Autodesk Inventor part; units mm, degrees
ref_plane "Work Plane1" through (0, 4.7752, 0) normal (0, -1, 0) x (1, 0, 0)
ref_plane "YZ Plane" through (0, 0, 0) normal (1, 0, 0) x (0, 1, 0)
ref_plane "XZ Plane" through (0, 0, 0) normal (0, 1, 0) x (-1, 0, 0)
sketch "Sketch2" plane through (0, 0, 0) normal (0, 1, 0) x (-1, 0, 0)
  line L0 (23, 23) -> (-23, 23)
  line L1 (-23, 23) -> (-23, -23)
  line L2 (-23, -23) -> (23, -23)
  line L3 (23, -23) -> (23, 23)
  line L4 (23, 23) -> (-23, -23) construction
  line L5 (-23, 23) -> (23, -23) construction
  circle A0 centre (19.05, -19.05) radius 1.8669
  line L6 (0, -32.2) -> (0, 32.2) construction
  line L7 (-32.2, 0) -> (32.2, 0) construction
  circle A1 centre (-19.05, -19.05) radius 1.8669
  circle A2 centre (19.05, 19.05) radius 1.8669
  circle A3 centre (-19.05, 19.05) radius 1.8669
  circle A4 centre (-5.1187, -2.6043) radius 2.794
  circle A5 centre (2.6043, 5.1187) radius 2.794
  circle A6 centre (10.6604, -10.6604) radius 2.413
  circle A7 centre (-10.6604, 10.6604) radius 2.413
  line L8 (2.6043, 5.1187) -> (-5.1187, -2.6043) construction
  point P0 (0, 0)
  point P1 (-1.2572, 1.2572)
  dimension "d4" = 46
  dimension "d5" = 46
  dimension "d8" = 38.1
  dimension "d11" = 38.1
  dimension "d14" = 3.7338
  dimension "d15" = 5.588
  dimension "d16" = 4.826
  dimension "d17" = 30.1521
  dimension "d18" = 15.0761
  dimension "d19" = 10.922
  dimension "d20" = 1.778
extrude "Extrusion1" add sketch "Sketch2" along normal blind 31.75 contours L3 L2 L1 L0 | A0 | A1 | A2 | A3 | A4 | A5 | A6 | A7
fillet "Fillet1" radius 6.35 4 edges at (-23, 15.875, 23) (-23, 15.875, -23) (23, 15.875, 23) (23, 15.875, -23)
ref_plane "Work Plane1" through (0, 4.7752, 0) normal (0, -1, 0) x (1, 0, 0)
sketch "Sketch3" plane through (0, 4.7752, 0) normal (0, -1, 0) x (1, 0, 0)
  circle A0 centre (0, 0) radius 19.812
  circle A1 centre (0, 0) radius 16.637
  line L0 (23, 16.65) -> (23, -16.65) construction
  line L1 (23, -5.9899) -> (15.9457, -4.746)
  line L2 (16.6073, -0.9939) -> (23, -2.1211)
  line L3 (16.6073, 0.9939) -> (23, 2.1211)
  line L4 (15.9457, 4.746) -> (23, 5.9899)
  line L5 (-36.211, 0) -> (36.9584, 0) construction
  line L6 (16.3842, -2.889) -> (23, -4.0555) construction
  line L7 (23, -2.1211) -> (23, 2.1211)
  line L8 (9.7506, -17.2465) -> (13.7792, -23)
  line L9 (16.65, -23) -> (-16.65, -23) construction
  line L10 (18.4303, -23) -> (12.8715, -15.0612)
  line L11 (15.0612, -12.8715) -> (23, -18.4303)
  line L12 (17.2465, -9.7506) -> (23, -13.7792)
  line L13 (0, 36.211) -> (0, -36.9584) construction
  line L14 (0, 0) -> (26.5056, -26.5056) construction
  line L15 (16.1048, -23) -> (11.3637, -16.229) construction
  arc A2 (18.4303, -23) -> (23, -18.4303) centre (21.1181, -21.1181) ccw
  line L16 (23, -13.7792) -> (23, -5.9899)
  line L17 (0.9939, 16.6073) -> (2.1211, 23)
  line L18 (5.9899, 23) -> (4.746, 15.9457)
  line L19 (2.1211, 23) -> (-2.1211, 23)
  line L20 (-0.9939, 16.6073) -> (-2.1211, 23)
  line L21 (-4.746, 15.9457) -> (-5.9899, 23)
  line L22 (13.7792, 23) -> (5.9899, 23)
  line L23 (9.7506, 17.2465) -> (13.7792, 23)
  line L24 (12.8715, 15.0612) -> (18.4303, 23)
  line L25 (23, 18.4303) -> (15.0612, 12.8715)
  line L26 (17.2465, 9.7506) -> (23, 13.7792)
  arc A3 (23, 18.4303) -> (18.4303, 23) centre (21.1181, 21.1181) ccw
  line L27 (-16.6073, 0.9939) -> (-23, 2.1211)
  line L28 (-23, 5.9899) -> (-15.9457, 4.746)
  line L29 (-23, 2.1211) -> (-23, -2.1211)
  line L30 (-16.6073, -0.9939) -> (-23, -2.1211)
  line L31 (-15.9457, -4.746) -> (-23, -5.9899)
  line L32 (-23, 13.7792) -> (-23, 5.9899)
  line L33 (-17.2465, 9.7506) -> (-23, 13.7792)
  line L34 (-15.0612, 12.8715) -> (-23, 18.4303)
  line L35 (-18.4303, 23) -> (-12.8715, 15.0612)
  line L36 (-9.7506, 17.2465) -> (-13.7792, 23)
  arc A4 (-18.4303, 23) -> (-23, 18.4303) centre (-21.1181, 21.1181) ccw
  line L37 (-0.9939, -16.6073) -> (-2.1211, -23)
  line L38 (-5.9899, -23) -> (-4.746, -15.9457)
  line L39 (-2.1211, -23) -> (2.1211, -23)
  line L40 (0.9939, -16.6073) -> (2.1211, -23)
  line L41 (4.746, -15.9457) -> (5.9899, -23)
  line L42 (-13.7792, -23) -> (-5.9899, -23)
  line L43 (-9.7506, -17.2465) -> (-13.7792, -23)
  line L44 (-12.8715, -15.0612) -> (-18.4303, -23)
  line L45 (-23, -18.4303) -> (-15.0612, -12.8715)
  line L46 (-17.2465, -9.7506) -> (-23, -13.7792)
  arc A5 (-23, -18.4303) -> (-18.4303, -23) centre (-21.1181, -21.1181) ccw
  line L47 (23, 5.9899) -> (23, 13.7792)
  line L48 (-5.9899, 23) -> (-13.7792, 23)
  line L49 (-23, -5.9899) -> (-23, -13.7792)
  line L50 (-23, -16.65) -> (-23, 16.65) construction
  line L51 (13.7792, -23) -> (5.9899, -23)
  point P0 (19.0898, 5.3004)
  dimension "d25" = 39.624
  dimension "d26" = 33.274
  dimension "d27" = 3.81
  dimension "d28" = 3.81
  dimension "d29" = 20
  dimension "d30" = 45
  dimension "d31" = 3.81
  dimension "d32" = 3.81
  dimension "d33" = 20
  dimension "d41" = 360
extrude "Extrusion2" cut sketch "Sketch3" against normal blind 31.75 contours A0 L4 A1 L18 | L26 L47 L4 A0 | A0 L24 A3 L25 | L3 L7 L2 A0 | A0 L2 A1 L3 | A1 | A0 L18 L22 L23 | A1 L20 A0 L17 | A0 L20 L19 L17 | L1 L16 L12 A0 | A0 L41 A1 L1 | A1 L28 A0 L21 | A0 L36 L48 L21 | L11 A2 L10 A0 | L40 A0 L37 A1 | A0 L8 L51 L41 | A1 L30 A0 L27 | L28 L32 L33 A0 | A0 L34 A4 L35 | L40 L39 L37 A0 | A0 L30 L29 L27 | L38 A0 L31 A1 | L38 L42 L43 A0 | A0 L46 L49 L31 | L44 A5 L45 A0
extrude "Extrusion3" cut sketch "Sketch2" along normal through all contours A0 | A1 | A2 | A3 | A4 | A5 | A6 | A7
equation "\"d18\" = 0.5 * d17"
equation "\"d28\" = d27"
equation "\"d31\" = d27"
equation "\"d32\" = d27"
properties part number "680-125K" material "Aluminum-5052"
The model under review builds one solid part; all positions refer to its coordinate system, in mm. A direction names the side the tool comes from. Round coordinates to 2 decimals unless told otherwise and drop trailing zeros. Order: outer loops, then holes, each group sorted by start corner. A loop starts at its lowest first (then second) coordinate and runs counter-clockwise, first axis right, second up. Notation, with made-up numbers: (57.5, 1) -> (101.5, 1) arc R5 cw to (101.5, 7) -> close; hole circle Ø6 at (16.25, 81). An arc over 180 degrees is marked (long way). One line per item, written item: value. Start each with the question number.
Q1. Take a section at D-D (x = -11). Write out the cut boundary in (y, z), and give its area (3 significant figures).
Q2. Machinability: for faces 4 (the face through (-5.377, 18.074, -19.522)), 5 (the face through (-11.737, 18.074, 20.083)), 6 (the face through (19.76, 18.07, -1.55)), which of the approach directions +Z, -Z, +X, -X, +Y, -Y give a long, thin tool a straight path to every point of the face, cutting with its end or side? Answer none if there is none.
Q3. Take a section at A-A (x = 19.05). Write out the cut boundary in (y, z).
Q4. Wall thickness on line 1 (X direction, y = 2, z = -19); line 2 (Z direction, x = -17.5, y = 22); line 3 (Z direction, x = -19, y = 25): over which ranges is each line inside the solid? List them lowest first.
Q5. Take a section at B-B (z = 7). Write out the cut boundary in (x, y).
Q6. Take a section at C-C (z = 19.05). Write out the cut boundary in (x, y), and give its area (3 significant figures).
Q7. Clearance check with a flat-ended pin moving along its axis: pin 1 Ø7.5 at (x, z) = (-10.66, -10.66) entering from +Y. State where the tip first meets the part, or that it passes through.
Q8. Mouldability with a two-part tool opening along X and no side actions: class faces 1 (the face through (-17.13, 12.57, -22.98)), 2 (the face through (-16.21, 18.07, 11.39)), 3 (the face through (17.13, 12.57, 22.98)) as released by +X, released by -X, zero draft, split by the parting line, or undercut.
Reported:
1. outline: (0, -23) -> (4.78, -23) -> (4.78, -19.03) -> (31.75, -19.03) -> (31.75, -16.48) -> (4.78, -16.48) -> (4.78, -13.05) -> (0, -13.05) -> close; (0, -8.27) -> (4.78, -8.27) -> (4.78, 16.48) -> (31.75, 16.48) -> (31.75, 19.03) -> (4.78, 19.03) -> (4.78, 23) -> (0, 23) -> close
1. area: 335 mm2
2. face 4: +Y
2. face 5: +Z, +Y
2. face 6: +X, +Y
3. outline: (0, -22.53) -> (4.78, -22.53) -> (4.78, -20.92) -> (0, -20.92) -> close; (0, -17.18) -> (4.78, -17.18) -> (4.78, -15.66) -> (31.75, -15.66) -> (31.75, -11.01) -> (4.78, -11.01) -> (4.78, -5.29) -> (31.75, -5.29) -> (31.75, -1.42) -> (4.78, -1.42) -> (4.78, 1.42) -> (31.75, 1.42) -> (31.75, 5.29) -> (4.78, 5.29) -> (4.78, 11.01) -> (31.75, 11.01) -> (31.75, 15.66) -> (4.78, 15.66) -> (4.78, 17.18) -> (0, 17.18) -> close; (0, 20.92) -> (4.78, 20.92) -> (4.78, 22.53) -> (0, 22.53) -> close
4. line 1: x = -22.55 to -20.92, -17.18 to 17.18, 20.92 to 22.55
4. line 2: z = -22.94 to -21.67, -14.58 to -9.93, -5.02 to -1.15, 1.15 to 5.02, 9.93 to 14.58, 21.67 to 22.94
4. line 3: z = -15.63 to -10.98, -5.28 to -1.42, 1.42 to 5.28, 10.98 to 15.63
5. outline: (-23, 0) -> (-4.67, 0) -> (-4.67, 4.78) -> (-23, 4.78) -> close; (-0.54, 0) -> (23, 0) -> (23, 4.78) -> (-0.54, 4.78) -> close
6. outline: (-22.53, 0) -> (-20.92, 0) -> (-20.92, 4.78) -> (-22.53, 4.78) -> close; (-17.18, 0) -> (17.18, 0) -> (17.18, 4.78) -> (15.66, 4.78) -> (15.66, 31.75) -> (11.01, 31.75) -> (11.01, 4.78) -> (5.29, 4.78) -> (5.29, 31.75) -> (1.42, 31.75) -> (1.42, 4.78) -> (-1.42, 4.78) -> (-1.42, 31.75) -> (-5.29, 31.75) -> (-5.29, 4.78) -> (-11.01, 4.78) -> (-11.01, 31.75) -> (-15.66, 31.75) -> (-15.66, 4.78) -> (-17.18, 4.78) -> close; (20.92, 0) -> (22.53, 0) -> (22.53, 4.78) -> (20.92, 4.78) -> close
6. area: 639 mm2
7. pin 1: stops at y = 4.78
8. face 1: released by -X
8. face 2: undercut
8. face 3: released by +X
